Geometry: final body of the model. Coordinates: model frame, mm. Face numbers are marked on the shaded views. A direction names the side the tool comes from. Give positions to 0.01 mm unless a question says otherwise; leave off trailing zeros. Loops run counter-clockwise (first coordinate to the right, second up) from the corner with the lowest first, then second, coordinate; pieces in that order, holes last. Notation, with made-up numbers: (-15, -22.5) - (33, -22.5) arc R26 cw to (33, -7.5) - close; hole circle Ø1 at (-6, -30.5). An arc over 180 degrees is marked (long way). Use one line per item in the form item = value.
```python
from build123d import *

# Parameters (mm, degrees)
SKETCH1_W                      = 152.4
SKETCH1_H                      = 101.6
BASE_FLANGE1_DEPTH             = 2.286
EDGE_FLANGE1_DEPTH             = 152.4
EDGE_FLANGE2_DEPTH             = 152.4
SKETCH14_W                     = 36.50996
SKETCH14_H                     = 46.482
CUT_EXTRUDE1_DEPTH             = 96.335271964
EDGE_FLANGE3_START             = 38.54704
EDGE_FLANGE3_DEPTH             = 37.65296
EDGE_FLANGE3_2_DEPTH           = 1.143
EDGE_FLANGE3_START_2           = 39.69004
EDGE_FLANGE3_3_DEPTH           = 36.50996
EDGE_FLANGE4_START             = 38.54704
EDGE_FLANGE4_DEPTH             = 37.65296
EDGE_FLANGE4_2_DEPTH           = 1.143
EDGE_FLANGE4_START_2           = 39.69004
EDGE_FLANGE4_3_DEPTH           = 36.50996
CUT_EXTRUDE3_REACH             = 112.14
SKETCH22_R                     = 3.3734375
CUT_EXTRUDE3_DIRECTION_2_REACH = 112.14
EDGE_FLANGE5_STRIP_W           = 10.6172
EDGE_FLANGE5_STRIP_H           = 2.286
EDGE_FLANGE5_STRIP_CUT_DEPTH   = 36.50996
EDGE_FLANGE5_DEPTH             = 36.50996
EDGE_FLANGE6_STRIP_W           = 10.6172
EDGE_FLANGE6_STRIP_H           = 2.286
EDGE_FLANGE6_STRIP_CUT_DEPTH   = 36.50996
EDGE_FLANGE6_DEPTH             = 36.50996
EDGE_FLANGE7_STRIP_W           = 10.6172
EDGE_FLANGE7_STRIP_H           = 2.286
EDGE_FLANGE7_STRIP_CUT_DEPTH   = 152.4
EDGE_FLANGE7_DEPTH             = 152.4
EDGE_FLANGE8_STRIP_W           = 10.6172
EDGE_FLANGE8_STRIP_H           = 2.286
EDGE_FLANGE8_STRIP_CUT_DEPTH   = 152.4
EDGE_FLANGE8_DEPTH             = 152.4
SKETCH35_W                     = 1.524
SKETCH35_H                     = 54.8132
CUT_EXTRUDE4_DEPTH             = 96.335271964


# Read off the part's stored shape, not the designer's step: Edge-Flange3, Edge-Flange4
# Sheet-metal steps are written as plain solids
with BuildPart() as part:
    # Sketch1 → Base-Flange1 (new body)
    with BuildSketch(Plane.XY):
        Rectangle(SKETCH1_W, SKETCH1_H)
    extrude(amount=-BASE_FLANGE1_DEPTH)

    # Edge-Flange1 section (across the edge) → Edge-Flange1 (add)
    with BuildSketch(Plane(origin=(-76.2, 51.5366, -2.286), x_dir=(0, -1, 0), z_dir=(1, 0, 0))):
        with BuildLine():
            Line((-2.286, 0.7366), (-2.286, 17.3482))
            Line((-2.286, 17.3482), (0, 17.3482))
            Line((0, 17.3482), (0, 0.7366))
            ThreePointArc((0, 0.7366), (0.215745145, 0.215745145), (0.7366, 0))
            Line((0.7366, 0), (0.7366, -2.286))
            ThreePointArc((0.7366, -2.286), (-1.400700957, -1.400700957), (-2.286, 0.7366))
        make_face()
    extrude(amount=EDGE_FLANGE1_DEPTH)

    # Edge-Flange2 section (across the edge) → Edge-Flange2 (add)
    with BuildSketch(Plane(origin=(76.2, -51.5366, -2.286), x_dir=(0, 1, 0), z_dir=(-1, 0, 0))):
        with BuildLine():
            Line((-2.286, 0.7366), (-2.286, 17.3482))
            Line((-2.286, 17.3482), (0, 17.3482))
            Line((0, 17.3482), (0, 0.7366))
            ThreePointArc((0, 0.7366), (0.215745145, 0.215745145), (0.7366, 0))
            Line((0.7366, 0), (0.7366, -2.286))
            ThreePointArc((0.7366, -2.286), (-1.400700957, -1.400700957), (-2.286, 0.7366))
        make_face()
    extrude(amount=EDGE_FLANGE2_DEPTH)

    # Sketch14 → Cut-Extrude1 (cut, through all)
    with BuildSketch(Plane.XY):
        with Locations((57.94502, 0)):
            Rectangle(SKETCH14_W, SKETCH14_H)
    extrude(amount=-CUT_EXTRUDE1_DEPTH, mode=Mode.SUBTRACT)

    # Edge-Flange3 outline → Edge-Flange3 (cut)
    with BuildSketch(Plane.YZ.offset(EDGE_FLANGE3_START)):
        with BuildLine():
            ThreePointArc((-26.2636, 0), (-24.404882216, -0.639056638), (-23.332127469, -2.286))
            Line((-23.332127469, -2.286), (-23.241, -2.286))
            Line((-23.241, -2.286), (-23.241, 0))
            Line((-23.241, 0), (-26.2636, 0))
        make_face()
    extrude(amount=EDGE_FLANGE3_DEPTH, mode=Mode.SUBTRACT)

    # Edge-Flange3 2 outline → Edge-Flange3 2 (cut)
    with BuildSketch(Plane.YZ.offset(EDGE_FLANGE3_START)):
        with BuildLine():
            Line((-27.4066, -2.286), (-23.332127469, -2.286))
            ThreePointArc((-23.332127469, -2.286), (-24.404882216, -0.639056638), (-26.2636, 0))
            Line((-26.2636, 0), (-27.4066, 0))
            Line((-27.4066, 0), (-27.4066, -2.286))
        make_face()
    extrude(amount=EDGE_FLANGE3_2_DEPTH, mode=Mode.SUBTRACT)

    # Edge-Flange3 3 outline → Edge-Flange3 3 (add)
    with BuildSketch(Plane.YZ.offset(EDGE_FLANGE3_START_2)):
        with BuildLine():
            Line((-25.527, -19.6342), (-23.241, -19.6342))
            Line((-23.241, -19.6342), (-23.241, -3.0226))
            ThreePointArc((-23.241, -3.0226), (-23.263868376, -2.651492275), (-23.332127469, -2.286))
            Line((-23.332127469, -2.286), (-26.2636, -2.286))
            ThreePointArc((-26.2636, -2.286), (-25.742745145, -2.501745145), (-25.527, -3.0226))
            Line((-25.527, -3.0226), (-25.527, -19.6342))
        make_face()
    extrude(amount=EDGE_FLANGE3_3_DEPTH)

    # Edge-Flange4 outline → Edge-Flange4 (cut)
    with BuildSketch(Plane.YZ.offset(EDGE_FLANGE4_START)):
        with BuildLine():
            Line((23.241, -2.286), (23.332127469, -2.286))
            ThreePointArc((23.332127469, -2.286), (24.404882216, -0.639056638), (26.2636, 0))
            Line((26.2636, 0), (23.241, 0))
            Line((23.241, 0), (23.241, -2.286))
        make_face()
    extrude(amount=EDGE_FLANGE4_DEPTH, mode=Mode.SUBTRACT)

    # Edge-Flange4 2 outline → Edge-Flange4 2 (cut)
    with BuildSketch(Plane.YZ.offset(EDGE_FLANGE4_START)):
        with BuildLine():
            Line((23.332127469, -2.286), (27.4066, -2.286))
            Line((27.4066, -2.286), (27.4066, 0))
            Line((27.4066, 0), (26.2636, 0))
            ThreePointArc((26.2636, 0), (24.404882216, -0.639056638), (23.332127469, -2.286))
        make_face()
    extrude(amount=EDGE_FLANGE4_2_DEPTH, mode=Mode.SUBTRACT)

    # Edge-Flange4 3 outline → Edge-Flange4 3 (add)
    with BuildSketch(Plane.YZ.offset(EDGE_FLANGE4_START_2)):
        with BuildLine():
            Line((23.241, -19.6342), (25.527, -19.6342))
            Line((25.527, -19.6342), (25.527, -3.0226))
            ThreePointArc((25.527, -3.0226), (25.742745145, -2.501745145), (26.2636, -2.286))
            Line((26.2636, -2.286), (23.332127469, -2.286))
            ThreePointArc((23.332127469, -2.286), (23.263868376, -2.651492275), (23.241, -3.0226))
            Line((23.241, -3.0226), (23.241, -19.6342))
        make_face()
    extrude(amount=EDGE_FLANGE4_3_DEPTH)

    # Cut-Extrude3: up to this face of the body (flat: up to its plane)
    cut_extrude3_end = Plane(part.part.faces().sort_by_distance((57.94502, -25.527, -11.3284))[0])
    # Sketch22 → Cut-Extrude3 (cut, up to the picked face)
    with BuildSketch(Plane(origin=(0, -23.241, 0), x_dir=(1, 0, 0), z_dir=(0, 1, 0)), mode=Mode.PRIVATE) as cut_extrude3_sk1:
        with Locations(Location((57.94502, 10.7442, 0), (0, 0, 270))):
            Circle(SKETCH22_R)
    cut_extrude3_tool1 = split(extrude(cut_extrude3_sk1.sketch, amount=-CUT_EXTRUDE3_REACH, mode=Mode.PRIVATE), bisect_by=cut_extrude3_end, keep=Keep.BOTH, mode=Mode.PRIVATE)
    add(cut_extrude3_tool1.solids().sort_by(Axis((57.94502, -23.241, -10.7442), (0, -1, 0)))[0], mode=Mode.SUBTRACT)

    # Cut-Extrude3 direction 2: up to this face of the body (flat: up to its plane)
    cut_extrude3_direction_2_end = Plane(part.part.faces().sort_by_distance((57.94502, 25.527, -11.3284))[0])
    # Sketch22 → Cut-Extrude3 direction 2 (cut, up to the picked face)
    with BuildSketch(Plane(origin=(0, -23.241, 0), x_dir=(1, 0, 0), z_dir=(0, 1, 0)), mode=Mode.PRIVATE) as cut_extrude3_direction_2_sk1:
        with Locations(Location((57.94502, 10.7442, 0), (0, 0, 270))):
            Circle(SKETCH22_R)
    cut_extrude3_direction_2_tool1 = split(extrude(cut_extrude3_direction_2_sk1.sketch, amount=CUT_EXTRUDE3_DIRECTION_2_REACH, mode=Mode.PRIVATE), bisect_by=cut_extrude3_direction_2_end, keep=Keep.BOTH, mode=Mode.PRIVATE)
    add(cut_extrude3_direction_2_tool1.solids().sort_by(Axis((57.94502, -23.241, -10.7442), (0, 1, 0)))[0], mode=Mode.SUBTRACT)

    # Edge-Flange5 strip (across the edge) → Edge-Flange5 strip cut (cut)
    with BuildSketch(Plane(origin=(39.69004, -25.527, -19.6342), x_dir=(0, 0, 1), z_dir=(1, 0, 0))):
        with Locations((-2.286, -1.143)):
            Rectangle(EDGE_FLANGE5_STRIP_W, EDGE_FLANGE5_STRIP_H)
    extrude(amount=EDGE_FLANGE5_STRIP_CUT_DEPTH, mode=Mode.SUBTRACT)

    # Edge-Flange5 section (across the edge) → Edge-Flange5 (add)
    with BuildSketch(Plane(origin=(39.69004, -25.527, -19.6342), x_dir=(0, 0, 1), z_dir=(1, 0, 0))):
        with BuildLine():
            Line((0, 0.7366), (0, 4.064))
            Line((0, 4.064), (2.286, 4.064))
            Line((2.286, 4.064), (2.286, 0.7366))
            ThreePointArc((2.286, 0.7366), (2.501745145, 0.215745145), (3.0226, 0))
            Line((3.0226, 0), (3.0226, -2.286))
            ThreePointArc((3.0226, -2.286), (0.885299043, -1.400700957), (0, 0.7366))
        make_face()
    extrude(amount=EDGE_FLANGE5_DEPTH)

    # Edge-Flange6 strip (across the edge) → Edge-Flange6 strip cut (cut)
    with BuildSketch(Plane(origin=(76.2, 25.527, -19.6342), x_dir=(0, 0, 1), z_dir=(-1, 0, 0))):
        with Locations((-2.286, -1.143)):
            Rectangle(EDGE_FLANGE6_STRIP_W, EDGE_FLANGE6_STRIP_H)
    extrude(amount=EDGE_FLANGE6_STRIP_CUT_DEPTH, mode=Mode.SUBTRACT)

    # Edge-Flange6 section (across the edge) → Edge-Flange6 (add)
    with BuildSketch(Plane(origin=(76.2, 25.527, -19.6342), x_dir=(0, 0, 1), z_dir=(-1, 0, 0))):
        with BuildLine():
            Line((0, 0.7366), (0, 4.064))
            Line((0, 4.064), (2.286, 4.064))
            Line((2.286, 4.064), (2.286, 0.7366))
            ThreePointArc((2.286, 0.7366), (2.501745145, 0.215745145), (3.0226, 0))
            Line((3.0226, 0), (3.0226, -2.286))
            ThreePointArc((3.0226, -2.286), (0.885299043, -1.400700957), (0, 0.7366))
        make_face()
    extrude(amount=EDGE_FLANGE6_DEPTH)

    # Edge-Flange7 strip (across the edge) → Edge-Flange7 strip cut (cut)
    with BuildSketch(Plane(origin=(76.2, -51.5366, -19.6342), x_dir=(0, 0, 1), z_dir=(-1, 0, 0))):
        with Locations((-2.286, -1.143)):
            Rectangle(EDGE_FLANGE7_STRIP_W, EDGE_FLANGE7_STRIP_H)
    extrude(amount=EDGE_FLANGE7_STRIP_CUT_DEPTH, mode=Mode.SUBTRACT)

    # Edge-Flange7 section (across the edge) → Edge-Flange7 (add)
    with BuildSketch(Plane(origin=(76.2, -51.5366, -19.6342), x_dir=(0, 0, 1), z_dir=(-1, 0, 0))):
        with BuildLine():
            Line((0, 0.7366), (0, 7.874))
            Line((0, 7.874), (2.286, 7.874))
            Line((2.286, 7.874), (2.286, 0.7366))
            ThreePointArc((2.286, 0.7366), (2.501745145, 0.215745145), (3.0226, 0))
            Line((3.0226, 0), (3.0226, -2.286))
            ThreePointArc((3.0226, -2.286), (0.885299043, -1.400700957), (0, 0.7366))
        make_face()
    extrude(amount=EDGE_FLANGE7_DEPTH)

    # Edge-Flange8 strip (across the edge) → Edge-Flange8 strip cut (cut)
    with BuildSketch(Plane(origin=(-76.2, 51.5366, -19.6342), x_dir=(0, 0, 1), z_dir=(1, 0, 0))):
        with Locations((-2.286, -1.143)):
            Rectangle(EDGE_FLANGE8_STRIP_W, EDGE_FLANGE8_STRIP_H)
    extrude(amount=EDGE_FLANGE8_STRIP_CUT_DEPTH, mode=Mode.SUBTRACT)

    # Edge-Flange8 section (across the edge) → Edge-Flange8 (add)
    with BuildSketch(Plane(origin=(-76.2, 51.5366, -19.6342), x_dir=(0, 0, 1), z_dir=(1, 0, 0))):
        with BuildLine():
            Line((0, 0.7366), (0, 7.874))
            Line((0, 7.874), (2.286, 7.874))
            Line((2.286, 7.874), (2.286, 0.7366))
            ThreePointArc((2.286, 0.7366), (2.501745145, 0.215745145), (3.0226, 0))
            Line((3.0226, 0), (3.0226, -2.286))
            ThreePointArc((3.0226, -2.286), (0.885299043, -1.400700957), (0, 0.7366))
        make_face()
    extrude(amount=EDGE_FLANGE8_DEPTH)

    # Sketch35 → Cut-Extrude4 (cut, through all)
    with BuildSketch(Plane.XY):
        with Locations((38.92804, 0)):
            Rectangle(SKETCH35_W, SKETCH35_H)
    extrude(amount=-CUT_EXTRUDE4_DEPTH, mode=Mode.SUBTRACT)


solid = part.part
```
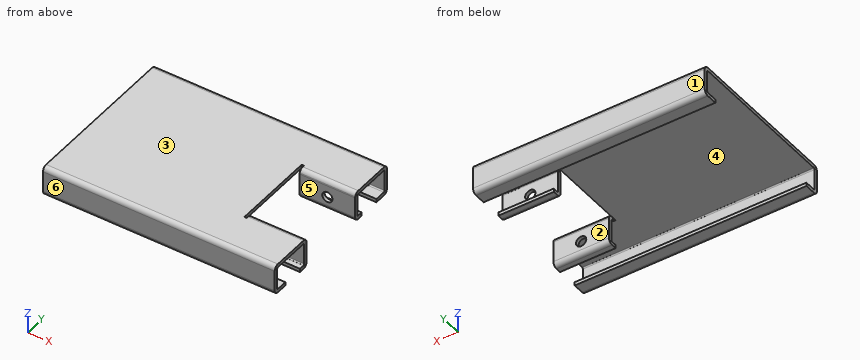
(1) Material intervals for L1, parallel to Y at x = 51, z = -13.5; L2, parallel to Y at x = -51, z = -15; L3, parallel to Z at x = 69.5, y = 27.5, sorted ascending. Write a range as from..to.
Solution:
L1 = -53.82..-51.54, -25.53..-23.24, 23.24..25.53, 51.54..53.82
L2 = -53.82..-51.54, 51.54..53.82
L3 = -19.63..-17.35, -2.29..0
(2) Cut plane D-D (y = -34). Return the cut outline in (x, z).
Solution:
outline = (-76.2, -2.29) - (76.2, -2.29) - (76.2, 0) - (-76.2, 0) - close
(3) Cut plane B-B (x = -42). Return the cut outline in (y, z).
Solution:
outline = (-53.82, -16.61) arc R3.02 ccw to (-50.8, -19.63) - (-43.66, -19.63) - (-43.66, -17.35) - (-50.8, -17.35) arc R0.74 cw to (-51.54, -16.61) - (-51.54, -3.02) arc R0.74 cw to (-50.8, -2.29) - (50.8, -2.29) arc R0.74 cw to (51.54, -3.02) - (51.54, -16.61) arc R0.74 cw to (50.8, -17.35) - (43.66, -17.35) - (43.66, -19.63) - (50.8, -19.63) arc R3.02 ccw to (53.82, -16.61) - (53.82, -3.02) arc R3.02 ccw to (50.8, 0) - (-50.8, 0) arc R3.02 ccw to (-53.82, -3.02) - close
(4) Cut plane A-A (z = -5.25). Return the cut outline in (x, y).
Solution:
outline = (-76.2, -53.82) - (76.2, -53.82) - (76.2, -51.54) - (-76.2, -51.54) - close; (-76.2, 51.54) - (76.2, 51.54) - (76.2, 53.82) - (-76.2, 53.82) - close; (39.69, -25.53) - (76.2, -25.53) - (76.2, -23.24) - (39.69, -23.24) - close; (39.69, 23.24) - (76.2, 23.24) - (76.2, 25.53) - (39.69, 25.53) - close
(5) Pin query (flat end, axial travel): P1, Ø1.1, axis at y = -10, z = -1.5, coming from the +X side; P2, Ø3, axis at y = 19.5, z = -4.5, coming from the +X side; P3, Ø5, axis at y = 27, z = -9, coming from the -X side; P4, Ø1.1, axis at x = 33.5, z = -18, coming from the +Y side. Return the tip coordinate at first contact, or that it passes through.
Solution:
P1 = 38.17
P2 = through
P3 = 39.69
P4 = 53.7
(6) Pull-direction query (Y, two-part tool) for the marked faces 3, 4, 5 and 6; classes: released by +Y, released by -Y, zero draft, split by the parting line, or undercut.
Solution:
face_3 = zero draft
face_4 = undercut
face_5 = undercut
face_6 = released by -Y
(7) Cut plane C-C (y = -2). Return the cut outline in (x, z), plus the area to 3 significant figures.
Solution:
outline = (-76.2, -2.29) - (38.17, -2.29) - (38.17, 0) - (-76.2, 0) - close
area = 261 mm2
(8) Access query for the marked faces 1 and 2. Directions: +Z, -Z, +X, -X, +Y, -Y. A direction counts if a zero-diameter tool reaches every point of the face in a straight line with its end or side. Return the directions, or none.
Solution:
face_1 = +Z, -Z, +X, -X, +Y
face_2 = +Z, -Z, +X, -X
